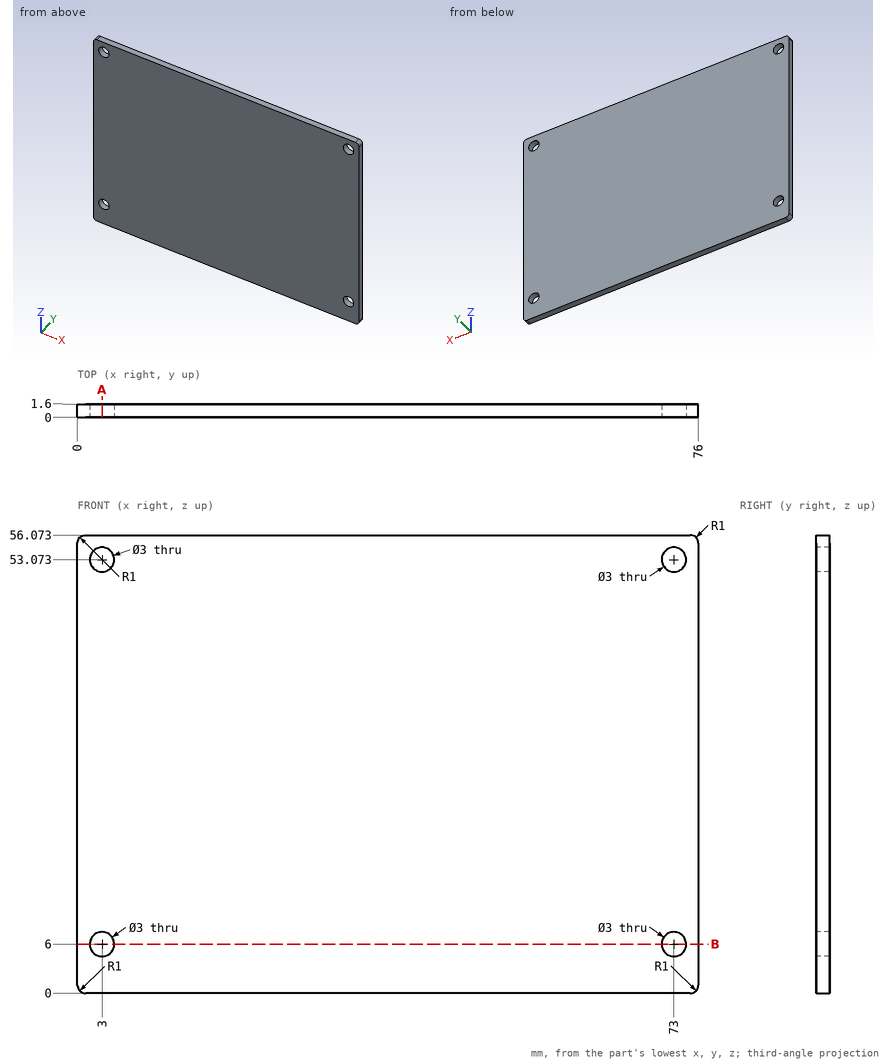
Input: dimensioned drawing with shaded views. Units: mm. Origin: part minimum x, y, z. Round coordinates to 2 decimals unless told otherwise and drop trailing zeros. Loops run counter-clockwise (first coordinate to the right, second up) from the corner with the lowest first, then second, coordinate; pieces in that order, holes last. Notation, with made-up numbers: M -36,0.25 L 18,0.25 A9 cw 18,7.25 Z; hole C 52,-20.75 d4. An arc over 180 degrees is marked long. One line per question, with ' | ' between items.
(1) Material intervals for line 1 along Z through (x, y) = (3, 0.5); line 2 along X through (y, z) = (0.8, 6); line 3 along X through (y, z) = (0.55, 5.5), sorted ascending. Write a range as from..to.
Check result:
line 1: z = 0..4.5, 7.5..51.57, 54.57..56.07 | line 2: x = 0..1.5, 4.5..71.5, 74.5..76 | line 3: x = 0..1.59, 4.41..71.59, 74.41..76
(2) Cut plane A-A on x = 3. Return the cut outline in (y, z), plus the area to 3 significant figures.
Check result:
outline: M 0,0 L 1.6,0 L 1.6,4.5 L 0,4.5 Z; M 0,7.5 L 1.6,7.5 L 1.6,51.57 L 0,51.57 Z; M 0,54.57 L 1.6,54.57 L 1.6,56.07 L 0,56.07 Z | area: 80.1 mm2
(3) Cut plane B-B on z = 6. Return the cut outline in (x, y), plus the area to 3 significant figures.
Check result:
outline: M 0,0 L 1.5,0 L 1.5,1.6 L 0,1.6 Z; M 4.5,0 L 71.5,0 L 71.5,1.6 L 4.5,1.6 Z; M 74.5,0 L 76,0 L 76,1.6 L 74.5,1.6 Z | area: 112 mm2
(4) Contact query for a flat-ended pin moving along its axis: P1, Ø5, axis at x = 3, z = 53.073, coming from the -Y side. Output: stop coordinate, or through.
Check result:
P1: stops at y = 0
